Job drawing, mm, ordinate dimensions from the low corner. One solid piece. Coordinates: 2 decimals unless noted, no trailing zeros. Write each loop counter-clockwise with the first axis right and the second up, starting at its lowest first coordinate (ties: lowest second). Pieces come first, ordered by that corner, then holes. Notation, with made-up numbers: (83, 81) -> (116, 81) arc R29 ccw to (116, 108) -> close; hole circle Ø4 at (47, -34.5). An arc over 180 degrees is marked (long way). Answer as a JSON object with one key per item and string values. Group by question number.
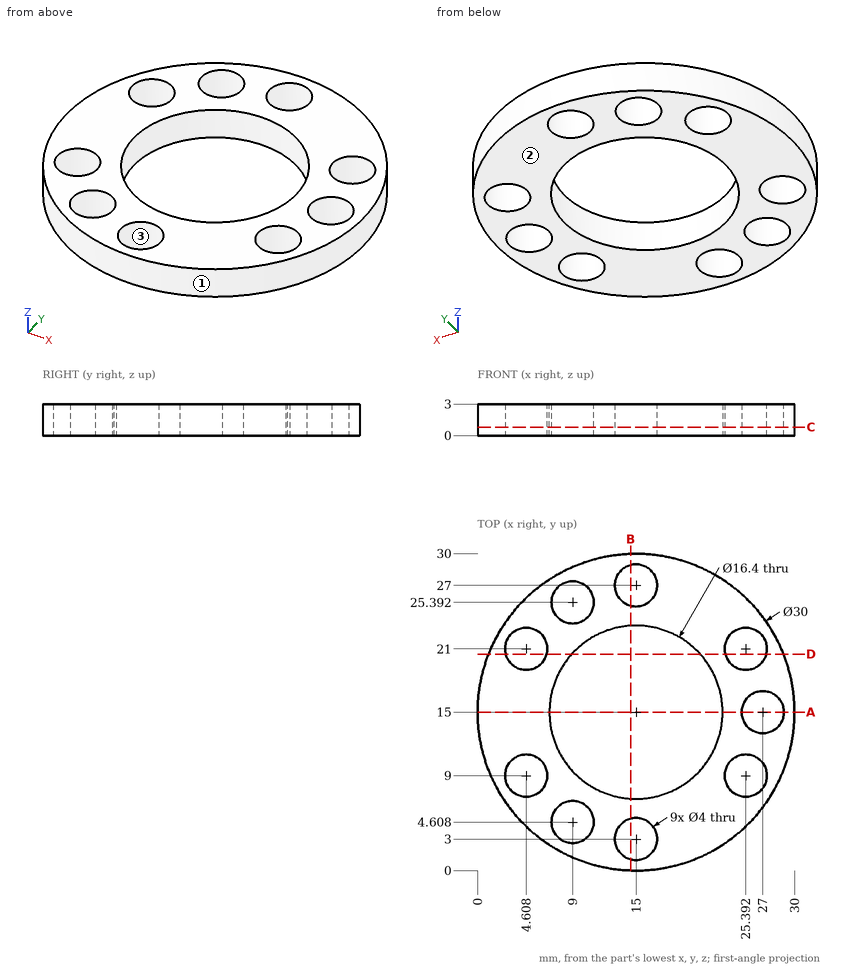
(1) Pin check, flat tip, straight feed: pin 1 (1.5 mm diameter, centred on x = 19, z = 2, fed in from +Y). Stop position of the tip, or through.
(2) Wall check: probe 1 along Y at (x, z) = (15, 1.45); probe 2 along Y at (x, z) = (9, 1.65); probe 3 along X at (y, z) = (8.5, 1.65) (1 decimal). Give the ranges that are in metal, low to high.
(3) Pull direction X, two halves, no side cores. Call the marked faces 1, 2 and 3: released by +X, released by -X, zero draft, split by the parting line, or undercut.
(4) Cut at C-C on z = 0.8. Give the number of separate pieces and of enclosed holes in the cut face.
(5) Cut at A-A on y = 15. List the corners of the cut face in (x, z), plus the area to 3 significant figures.
(6) Cut at B-B on x = 14.5. List the corners of the cut face in (y, z) (1 decimal).
(7) Cut at D-D on y = 20.5. List the corners of the cut face in (x, z) (1 decimal), plus the area to 3 significant figures.
Results found:
{
 "1": {"pin 1": "stops at y = 29.64"},
 "2": {"probe 1": "y = 0 to 1, 5 to 6.8, 23.2 to 25, 29 to 30", "probe 2": "y = 1.25 to 2.61, 6.61 to 9.41, 20.59 to 23.39, 27.39 to 28.75", "probe 3": "x = 1.5 to 2.7, 6.5 to 10, 20 to 23.5, 27.3 to 28.5"},
 "3": {"face 1": "split by the parting line", "face 2": "zero draft", "face 3": "undercut"},
 "4": {"separate pieces": "1", "enclosed holes": "10"},
 "5": {"outline": "(0, 0) -> (6.8, 0) -> (6.8, 3) -> (0, 3) -> close; (23.2, 0) -> (25, 0) -> (25, 3) -> (23.2, 3) -> close; (29, 0) -> (30, 0) -> (30, 3) -> (29, 3) -> close", "area": "28.8 mm²"},
 "6": {"outline": "(0, 0) -> (1.1, 0) -> (1.1, 3) -> (0, 3) -> close; (4.9, 0) -> (6.8, 0) -> (6.8, 3) -> (4.9, 3) -> close; (23.2, 0) -> (25.1, 0) -> (25.1, 3) -> (23.2, 3) -> close; (28.9, 0) -> (30, 0) -> (30, 3) -> (28.9, 3) -> close"},
 "7": {"outline": "(1, 0) -> (2.7, 0) -> (2.7, 3) -> (1, 3) -> close; (6.5, 0) -> (8.9, 0) -> (8.9, 3) -> (6.5, 3) -> close; (21.1, 0) -> (23.5, 0) -> (23.5, 3) -> (21.1, 3) -> close; (27.3, 0) -> (29, 0) -> (29, 3) -> (27.3, 3) -> close", "area": "24.0 mm²"}
}
